Can you work these out from the model? Positions are in its coordinate system, mm. A direction names the side the tool comes from. Round coordinates to 2 decimals unless told otherwise and drop trailing zeros. Write each loop counter-clockwise with the first axis right and the second up, starting at its lowest first coordinate (ties: lowest second). Pieces come first, ordered by that corner, then holes.
Q1. If we section it at D-D (x = 7.25): Please give me the cut outline in (y, z).
Q2. For faces 4 (the flat face through (1, 10, 5.842)), 5 (the flat face through (-2.75, 0, 5)), 6 (the flat face through (4, 0, 10.287)), which set-ups out of +Z, -Z, +X, -X, +Y, -Y let a thin tool reach every point of the face, with its end or its side?
Q3. If we section it at A-A (y = 0): Please give me the cut outline in (x, z) (3 decimals).
Q4. Please list where these lines run through material, in increasing order: line 1 along Y through (x, z) = (0, 3.25) (3 decimals); line 2 along Y through (x, z) = (0, 6.5) (3 decimals); line 3 along Z through (x, y) = (-1.75, 9.5).
Q5. I'm going to push flat-ended pins straight in: pin 1 Ø3 at (y, z) = (8, 5) entering from -X; pin 2 Ø4 at (y, z) = (3, 6.5) entering from -X; pin 3 Ø4 at (y, z) = (3.5, 1.5) entering from +X. Where does each tip first touch, or does it pass through?
Q6. We'd pull the mould along Y, two halves only. Please class faces 1 (the cylindrical face through (3.073, -0.115, 5.216)), 2 (the flat face through (2.3, -2.3, 0)), 3 (the cylindrical face through (9.014, -2.839, 8.033)): +Y half, -Y half, draft (parallel to the pull), parting line (faces both ways), or undercut.
Q7. If we section it at C-C (z = 7.5): Please give me the cut outline in (x, y) (3 decimals), plus the area to 3 significant figures.
Q8. If we section it at B-B (x = 0): Please give me the cut outline in (y, z) (3 decimals).
Autodesk Inventor part; units mm, degrees
ref_plane "YZ Plane" through (0, 0, 0) normal (1, 0, 0) x (0, 1, 0)
ref_plane "XZ Plane" through (0, 0, 0) normal (0, 1, 0) x (-1, 0, 0)
ref_plane "XY Plane" through (0, 0, 0) normal (0, 0, 1) x (1, 0, 0)
sketch "Sketch1" plane through (0, 0, 0) normal (0, 0, 1) x (1, 0, 0)
  circle A0 centre (0, 0) radius 10.85
  dimension "d0" = 21.7
extrude "Extrusion1" add sketch "Sketch1" along normal blind 5.842
sketch "Sketch2" plane through (0, 0, 5.842) normal (0, 0, 1) x (1, 0, 0)
  circle A0 centre (0, 0) radius 9.45
  dimension "d3" = 18.9
extrude "Extrusion2" add sketch "Sketch2" along normal blind 4.445
sketch "Sketch3" plane through (0, 0, 10.287) normal (0, 0, 1) x (1, 0, 0)
  circle A0 centre (0, 0) radius 3.075
  circle A1 centre (0, 0) radius 10.85 construction
  line L0 (-10.85, 0) -> (10.85, 0) construction
  circle A2 centre (0, 0) radius 9.45 construction
  line L1 (0, 9.45) -> (0, -9.45) construction
  line L2 (-2.75, 1.3759) -> (-2.75, -1.3759)
  dimension "d13" = 6.15
  dimension "d16" = 2.75
extrude "Extrusion3" cut sketch "Sketch3" against normal through all contours A0 L2 picked at (-0.8083, 0)
properties part number "wheel_mount"
A:
1. outline: (-8.07, 0) - (8.07, 0) - (8.07, 5.84) - (6.06, 5.84) - (6.06, 10.29) - (-6.06, 10.29) - (-6.06, 5.84) - (-8.07, 5.84) - close
2. face 4: +Z
2. face 5: +Z, -Z
2. face 6: +Z, +X, -X, +Y, -Y
3. outline: (-10.85, 0) - (-2.75, 0) - (-2.75, 10.287) - (-9.45, 10.287) - (-9.45, 5.842) - (-10.85, 5.842) - close; (3.075, 0) - (10.85, 0) - (10.85, 5.842) - (9.45, 5.842) - (9.45, 10.287) - (3.075, 10.287) - close
4. line 1: y = -10.85 to -3.075, 3.075 to 10.85
4. line 2: y = -9.45 to -3.075, 3.075 to 9.45
4. line 3: z = 0 to 5.84
5. pin 1: stops at x = -8.69
5. pin 2: stops at x = -10.79
5. pin 3: stops at x = 10.75
6. face 1: undercut
6. face 2: draft
6. face 3: parting line
7. outline: circle Ø18.9 at (0, 0); hole (-2.75, -1.376) arc R3.075 ccw (long way) to (-2.75, 1.376) - close
7. area: 251 mm2
8. outline: (-10.85, 0) - (-3.075, 0) - (-3.075, 10.287) - (-9.45, 10.287) - (-9.45, 5.842) - (-10.85, 5.842) - close; (3.075, 0) - (10.85, 0) - (10.85, 5.842) - (9.45, 5.842) - (9.45, 10.287) - (3.075, 10.287) - close
